```python
from build123d import *

# Parameters (mm, degrees)
F1_DEPTH = 5.9


with BuildPart() as f1:
    # F0 (on Top) → F1 (new body)
    with BuildSketch(Plane.XY):
        with BuildLine():
            Line((11.5, 0), (9.5, 0))
            ThreePointArc((9.5, 0), (9.1762953497, -2.4587809285), (8.227241336, -4.75))
            Line((8.227241336, -4.75), (9.9592921435, -5.75))
            ThreePointArc((9.9592921435, -5.75), (11.1081470023, -2.9764190187), (11.5, 0))
        make_face()
        with BuildLine():
            ThreePointArc((8.227241336, 4.75), (9.1762953497, 2.4587809285), (9.5, 0))
            Line((9.5, 0), (11.5, 0))
            ThreePointArc((11.5, 0), (11.1081470023, 2.9764190187), (9.9592921435, 5.75))
            Line((9.9592921435, 5.75), (8.227241336, 4.75))
        make_face()
        with BuildLine():
            ThreePointArc((0, 9.5), (4.75, 8.227241336), (8.227241336, 4.75))
            Line((8.227241336, 4.75), (9.9592921435, 5.75))
            ThreePointArc((9.9592921435, 5.75), (8.1317279836, 8.1317279836), (5.75, 9.9592921435))
            ThreePointArc((5.75, 9.9592921435), (2.9764190187, 11.1081470023), (0, 11.5))
            Line((0, 11.5), (0, 9.5))
        make_face()
        with BuildLine():
            Line((9.9592921435, -5.75), (8.227241336, -4.75))
            ThreePointArc((8.227241336, -4.75), (4.75, -8.227241336), (0, -9.5))
            Line((0, -9.5), (0, -11.5))
            ThreePointArc((0, -11.5), (2.9764190187, -11.1081470023), (5.75, -9.9592921435))
            ThreePointArc((5.75, -9.9592921435), (8.1317279836, -8.1317279836), (9.9592921435, -5.75))
        make_face()
        with BuildLine():
            Line((21.7644823154, 0), (11.5, 0))
            ThreePointArc((11.5, 0), (11.1081470023, -2.9764190187), (9.9592921435, -5.75))
            Line((9.9592921435, -5.75), (16.02146997, -9.25))
            ThreePointArc((16.02146997, -9.25), (20.0781480078, -5.1303927779), (25.6267837466, -3.5054491468))
            ThreePointArc((25.6267837466, -3.5054491468), (23.9098470955, -1.5167036662), (21.7644823154, 0))
        make_face()
        with BuildLine():
            ThreePointArc((21.7644823154, 0), (16.6322411577, 1.2934670156), (11.5, 0))
            Line((11.5, 0), (21.7644823154, 0))
        make_face()
        with BuildLine():
            ThreePointArc((-8.227241336, 4.75), (-4.75, 8.227241336), (0, 9.5))
            Line((0, 9.5), (0, 11.5))
            ThreePointArc((0, 11.5), (-2.9764190187, 11.1081470023), (-5.75, 9.9592921435))
            ThreePointArc((-5.75, 9.9592921435), (-8.1317279836, 8.1317279836), (-9.9592921435, 5.75))
            Line((-9.9592921435, 5.75), (-8.227241336, 4.75))
        make_face()
        with BuildLine():
            Line((0, -11.5), (0, -9.5))
            ThreePointArc((0, -9.5), (-4.75, -8.227241336), (-8.227241336, -4.75))
            Line((-8.227241336, -4.75), (-9.9592921435, -5.75))
            ThreePointArc((-9.9592921435, -5.75), (-8.1317279836, -8.1317279836), (-5.75, -9.9592921435))
            ThreePointArc((-5.75, -9.9592921435), (-2.9764190187, -11.1081470023), (0, -11.5))
        make_face()
        with BuildLine():
            Line((16.02146997, -9.25), (9.9592921435, -5.75))
            ThreePointArc((9.9592921435, -5.75), (8.1317279836, -8.1317279836), (5.75, -9.9592921435))
            ThreePointArc((5.75, -9.9592921435), (8.7759533757, -17.1498563505), (15.8491998862, -20.4407211685))
            ThreePointArc((15.8491998862, -20.4407211685), (14.4821244809, -14.8229898467), (16.02146997, -9.25))
        make_face()
        with BuildLine():
            Line((-9.9592921435, -5.75), (-8.227241336, -4.75))
            ThreePointArc((-8.227241336, -4.75), (-9.1762953497, -2.4587809285), (-9.5, 0))
            Line((-9.5, 0), (-11.5, 0))
            ThreePointArc((-11.5, 0), (-11.1081470023, -2.9764190187), (-9.9592921435, -5.75))
        make_face()
        with BuildLine():
            Line((-11.5, 0), (-9.5, 0))
            ThreePointArc((-9.5, 0), (-9.1762953497, 2.4587809285), (-8.227241336, 4.75))
            Line((-8.227241336, 4.75), (-9.9592921435, 5.75))
            ThreePointArc((-9.9592921435, 5.75), (-11.1081470023, 2.9764190187), (-11.5, 0))
        make_face()
        with BuildLine():
            Line((0, 18.5), (0, 11.5))
            ThreePointArc((0, 11.5), (2.9764190187, 11.1081470023), (5.75, 9.9592921435))
            ThreePointArc((5.75, 9.9592921435), (10.464234583, 16.1751267411), (9.7775838605, 23.9461703153))
            ThreePointArc((9.7775838605, 23.9461703153), (5.5960235268, 19.9533826246), (0, 18.5))
        make_face()
        with BuildLine():
            ThreePointArc((-5.75, 9.9592921435), (-2.9764190187, 11.1081470023), (0, 11.5))
            Line((0, 11.5), (0, 18.5))
            ThreePointArc((0, 18.5), (-5.5960235268, 19.9533826246), (-9.7775838605, 23.9461703153))
            ThreePointArc((-9.7775838605, 23.9461703153), (-10.464234583, 16.1751267411), (-5.75, 9.9592921435))
        make_face()
        with BuildLine():
            ThreePointArc((25.6267837466, -3.5054491468), (20.0781480078, -5.1303927779), (16.02146997, -9.25))
            Line((16.02146997, -9.25), (17.7535207776, -10.25))
            ThreePointArc((17.7535207776, -10.25), (21.5421151907, -6.6006897013), (26.6916116991, -5.5266324432))
            ThreePointArc((26.6916116991, -5.5266324432), (26.212648084, -4.4878813308), (25.6267837466, -3.5054491468))
        make_face()
        with BuildLine():
            Line((17.7535207776, -10.25), (16.02146997, -9.25))
            ThreePointArc((16.02146997, -9.25), (14.4821244809, -14.8229898467), (15.8491998862, -20.4407211685))
            ThreePointArc((15.8491998862, -20.4407211685), (16.9929432837, -20.4568784758), (18.1320099427, -20.3522975778))
            ThreePointArc((18.1320099427, -20.3522975778), (16.4874225591, -15.3556741558), (17.7535207776, -10.25))
        make_face()
        with BuildLine():
            Line((-16.02146997, -9.25), (-9.9592921435, -5.75))
            ThreePointArc((-9.9592921435, -5.75), (-11.1081470023, -2.9764190187), (-11.5, 0))
            Line((-11.5, 0), (-21.7644823154, 0))
            ThreePointArc((-21.7644823154, 0), (-23.9098470955, -1.5167036662), (-25.6267837466, -3.5054491468))
            ThreePointArc((-25.6267837466, -3.5054491468), (-20.0781480078, -5.1303927779), (-16.02146997, -9.25))
        make_face()
        with BuildLine():
            ThreePointArc((-5.75, -9.9592921435), (-8.1317279836, -8.1317279836), (-9.9592921435, -5.75))
            Line((-9.9592921435, -5.75), (-16.02146997, -9.25))
            ThreePointArc((-16.02146997, -9.25), (-14.8726151112, -12.0235809813), (-14.4807621135, -15))
            ThreePointArc((-14.4807621135, -15), (-14.8281174582, -17.8050877335), (-15.8491998862, -20.4407211685))
            ThreePointArc((-15.8491998862, -20.4407211685), (-8.7759533757, -17.1498563505), (-5.75, -9.9592921435))
        make_face()
        with BuildLine():
            Line((-21.7644823154, 0), (-11.5, 0))
            ThreePointArc((-11.5, 0), (-16.6322411577, 1.2934670156), (-21.7644823154, 0))
        make_face()
        with BuildLine():
            ThreePointArc((37.4807621135, -15), (33.9863616782, -6.7440702759), (25.6267837466, -3.5054491468))
            ThreePointArc((25.6267837466, -3.5054491468), (26.212648084, -4.4878813308), (26.6916116991, -5.5266324432))
            ThreePointArc((26.6916116991, -5.5266324432), (32.945066496, -8.5386948324), (35.4807621135, -15))
            ThreePointArc((35.4807621135, -15), (28.7813740446, -24.077806608), (18.1320099427, -20.3522975778))
            ThreePointArc((18.1320099427, -20.3522975778), (16.9929432837, -20.4568784758), (15.8491998862, -20.4407211685))
            ThreePointArc((15.8491998862, -20.4407211685), (28.785849847, -26.1526446553), (37.4807621135, -15))
        make_face()
        with BuildLine():
            ThreePointArc((-9.7775838605, 23.9461703153), (-5.5960235268, 19.9533826246), (0, 18.5))
            Line((0, 18.5), (0, 20.5))
            ThreePointArc((0, 20.5), (-5.0546926316, 21.956363857), (-8.5596017564, 25.8789300209))
            ThreePointArc((-8.5596017564, 25.8789300209), (-9.2197048003, 24.9447598066), (-9.7775838605, 23.9461703153))
        make_face()
        with BuildLine():
            Line((0, 20.5), (0, 18.5))
            ThreePointArc((0, 18.5), (5.5960235268, 19.9533826246), (9.7775838605, 23.9461703153))
            ThreePointArc((9.7775838605, 23.9461703153), (9.2197048003, 24.9447598066), (8.5596017564, 25.8789300209))
            ThreePointArc((8.5596017564, 25.8789300209), (5.0546926316, 21.956363857), (0, 20.5))
        make_face()
        with BuildLine():
            ThreePointArc((8.5596017564, 25.8789300209), (9.2197048003, 24.9447598066), (9.7775838605, 23.9461703153))
            ThreePointArc((9.7775838605, 23.9461703153), (11.0610174576, 26.8529549094), (11.5, 30))
            ThreePointArc((11.5, 30), (-3.1470450906, 41.0610174576), (-9.7775838605, 23.9461703153))
            ThreePointArc((-9.7775838605, 23.9461703153), (-9.2197048003, 24.9447598066), (-8.5596017564, 25.8789300209))
            ThreePointArc((-8.5596017564, 25.8789300209), (-2.1135022255, 39.2619170987), (9.5, 30))
            ThreePointArc((9.5, 30), (9.2619170987, 27.8864977745), (8.5596017564, 25.8789300209))
        make_face()
        with BuildLine():
            ThreePointArc((-14.4807621135, -15), (-14.8726151112, -12.0235809813), (-16.02146997, -9.25))
            Line((-16.02146997, -9.25), (-17.7535207776, -10.25))
            ThreePointArc((-17.7535207776, -10.25), (-16.8044667638, -12.5412190715), (-16.4807621135, -15))
            ThreePointArc((-16.4807621135, -15), (-16.9029555056, -17.8006119311), (-18.1320099427, -20.3522975778))
            ThreePointArc((-18.1320099427, -20.3522975778), (-16.9929432837, -20.4568784758), (-15.8491998862, -20.4407211685))
            ThreePointArc((-15.8491998862, -20.4407211685), (-14.8281174582, -17.8050877335), (-14.4807621135, -15))
        make_face()
        with BuildLine():
            Line((-17.7535207776, -10.25), (-16.02146997, -9.25))
            ThreePointArc((-16.02146997, -9.25), (-20.0781480078, -5.1303927779), (-25.6267837466, -3.5054491468))
            ThreePointArc((-25.6267837466, -3.5054491468), (-26.212648084, -4.4878813308), (-26.6916116991, -5.5266324432))
            ThreePointArc((-26.6916116991, -5.5266324432), (-21.5421151907, -6.6006897013), (-17.7535207776, -10.25))
        make_face()
        with BuildLine():
            ThreePointArc((-25.6267837466, -3.5054491468), (-35.9400542571, -20.75), (-15.8491998862, -20.4407211685))
            ThreePointArc((-15.8491998862, -20.4407211685), (-16.9929432837, -20.4568784758), (-18.1320099427, -20.3522975778))
            ThreePointArc((-18.1320099427, -20.3522975778), (-34.2080034495, -19.75), (-26.6916116991, -5.5266324432))
            ThreePointArc((-26.6916116991, -5.5266324432), (-26.212648084, -4.4878813308), (-25.6267837466, -3.5054491468))
        make_face()
    extrude(amount=F1_DEPTH)


solid = f1.part
```
The listing builds one solid part. Answer for the finished solid, in the listing's coordinates (mm). Coordinates: 2 decimals unless noted, no trailing zeros. Loops run counter-clockwise (first coordinate to the right, second up) from the corner with the lowest first, then second, coordinate; pieces in that order, holes last. Notation, with made-up numbers: M 4,57 L 59,57 A6 ccw 59,67 Z; hole C 41,11.25 d8. An arc over 180 degrees is marked long. Answer as CSV lines item,"result". Start each with the question number.
(1) The part is cut by section B-B (y = 37.5). Give the vertices of the cut face in (x, z), and give its area (3 significant figures).
(2) The part is cut by section C-C (y = -18). Give the vertices of the cut face in (x, z).
(3) Find the intervals of material crossed by L1, parallel to X at y = 30, z = 4.55; L2, parallel to Y at x = -8, z = 3.85; L3, parallel to Y at x = -3, z = 0.85, in increasing order. Write a range as [from, to].
(4) The part is cut by section D-D (z = 3.8). Give the vertices of the cut face in (x, y).
(5) The mould has two halves that part along Y. Classify faces 1 (the flat face through (0, -10, 5.9)), 2 (the cylindrical face through (-36.107, -20.451, 2.909)), 3 (the cylindrical face through (10.433, 16.068, 2.909)): pulls with the +Y half, pulls with the -Y half, needs draft (parallel to the pull), parting line crosses it, or undercut.
(6) Given pin 1 (3 mm diameter, centred on y = 0.5, z = 4, fed in from +X); pin 2 (3 mm diameter, centred on y = -10, z = 3, fed in from +X), each flat-ended and moving along its own axis, determine where each tip first touches the part or whether it passes through.
(7) The part is cut by section A-A (x = -28). Give the vertices of the cut face in (y, z), and give its area (3 significant figures).
Determined:
1,outline,"M -8.72,0 L -5.83,0 L -5.83,5.9 L -8.72,5.9 Z; M 5.83,0 L 8.72,0 L 8.72,5.9 L 5.83,5.9 Z"
1,area,"34.1 mm2"
2,outline,"M -37.08,0 L -34.99,0 L -34.99,5.9 L -37.08,5.9 Z; M -16.97,0 L -9.7,0 L -9.7,5.9 L -16.97,5.9 Z; M 9.7,0 L 16.97,0 L 16.97,5.9 L 9.7,5.9 Z; M 34.99,0 L 37.08,0 L 37.08,5.9 L 34.99,5.9 Z"
3,L1,"[-11.5, -9.5], [9.5, 11.5]"
3,L2,"[-16.25, -5.12], [5.12, 8.26], [11.81, 24.88], [35.12, 38.26]"
3,L3,"[-11.1, -9.01], [9.01, 20.99], [39.01, 41.1]"
4,outline,"M -25.63,-3.51 A11.5 ccw long -15.85,-20.44 A10.83 ccw -5.75,-9.96 A11.5 ccw 5.75,-9.96 A10.83 ccw 15.85,-20.44 A11.5 ccw long 25.63,-3.51 A10.83 ccw 11.5,0 A11.5 ccw 5.75,9.96 A10.83 ccw 9.78,23.95 A11.5 ccw long -9.78,23.95 A10.83 ccw -5.75,9.96 A11.5 ccw -11.5,0 A10.83 ccw Z; hole C -25.98,-15 d19; hole C 0,0 d19; hole C 0,30 d19; hole C 25.98,-15 d19"
5,face 1,"needs draft"
5,face 2,"parting line crosses it"
5,face 3,"undercut"
6,pin 1,"x = 23.3"
6,pin 2,"x = 36.94"
7,outline,"M -26.32,0 L -24.28,0 L -24.28,5.9 L -26.32,5.9 Z; M -5.72,0 L -3.68,0 L -3.68,5.9 L -5.72,5.9 Z"
7,area,"24.1 mm2"
